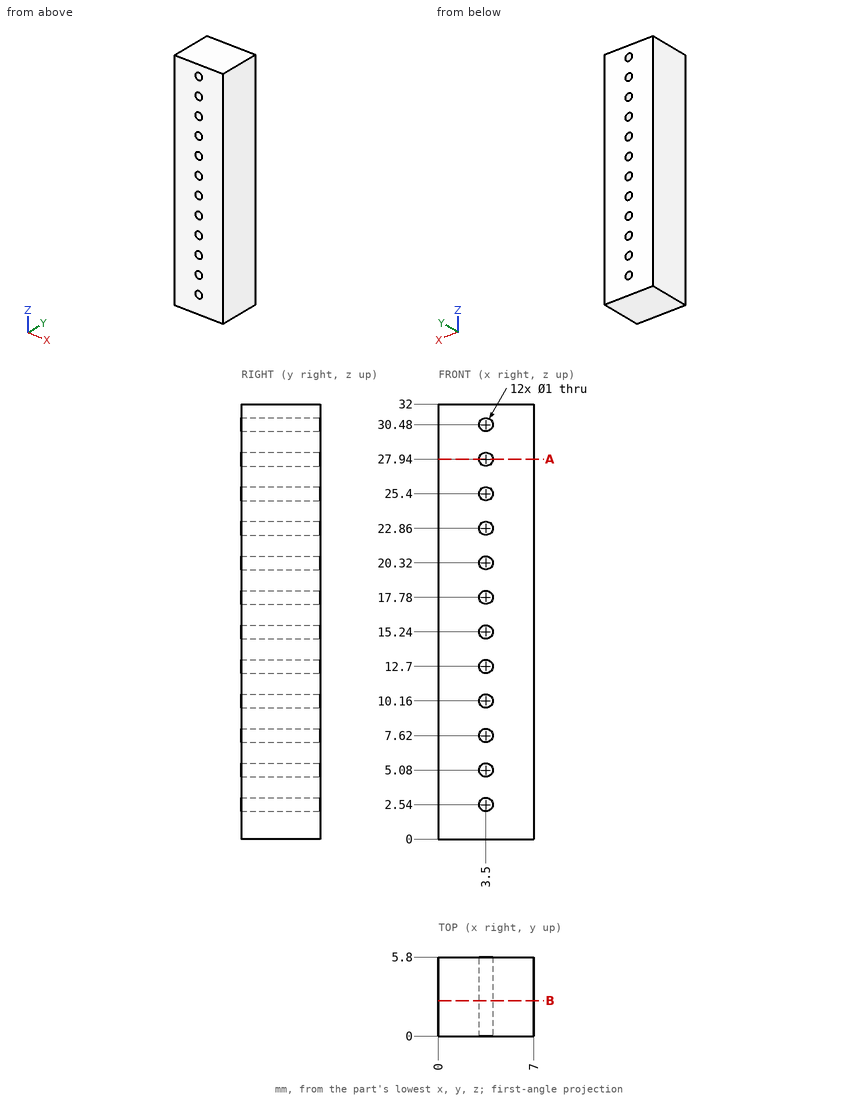
The drawing under review shows one solid part. Ordinate dimensions are in mm from its lowest x, y, z. Coordinates: 2 decimals unless noted, no trailing zeros. Write each loop counter-clockwise with the first axis right and the second up, starting at its lowest first coordinate (ties: lowest second). Pieces come first, ordered by that corner, then holes.
1) To check wall thickness, follow L1, parallel to X at y = 2.55, z = 10.16; L2, parallel to X at y = 3.75, z = 25. State the ranges of each line that lie inside material, in increasing order.
2) Add section B-B (y = 2.6). State how many separate pieces and enclosed holes the cut face has, plus the area to 3 significant figures.
3) Add section A-A (z = 27.94). Write out the cut boundary in (x, y), plus the area to 3 significant figures.
4) Insertion check: pin 1 (1.5 mm diameter, centred on x = 4.5, y = 3, fed in from -Z). The pin has a flat end and moves straight along its axis. Give the tip position at first contact, or say it passes through.
Check result:
1. L1: x = 0 to 3, 4 to 7
1. L2: x = 0 to 3.2, 3.8 to 7
2. separate pieces: 1
2. enclosed holes: 12
2. area: 215 mm2
3. outline: (0, 0) - (3, 0) - (3, 5.8) - (0, 5.8) - close; (4, 0) - (7, 0) - (7, 5.8) - (4, 5.8) - close
3. area: 34.8 mm2
4. pin 1: stops at z = 0
